Autodesk Inventor part; units mm, degrees
ref_plane "YZ Plane" through (0, 0, 0) normal (1, 0, 0) x (0, 1, 0)
ref_plane "XZ Plane" through (0, 0, 0) normal (0, 1, 0) x (-1, 0, 0)
ref_plane "XY Plane" through (0, 0, 0) normal (0, 0, 1) x (1, 0, 0)
sketch "Sketch1" plane through (0, 0, 0) normal (0, 1, 0) x (-1, 0, 0)
  line L0 (-43.5, 202.3853) -> (-0.5, 202.3853) construction
  line L1 (-0.5, 202.3853) -> (-0.5, 140.3853) construction
  line L2 (-0.5, 140.3853) -> (-43.5, 140.3853) construction
  line L3 (-43.5, 140.3853) -> (-43.5, 202.3853) construction
  line L4 (0, 112) -> (0, 260) construction
  line L5 (2.5, 205.3853) -> (-46.5, 205.3853) construction
  line L6 (-46.5, 205.3853) -> (-46.5, 137.3853) construction
  line L7 (-46.5, 137.3853) -> (2.5, 137.3853) construction
  line L8 (2.5, 137.3853) -> (2.5, 205.3853) construction
  line L9 (21.9355, 171.3853) -> (-82.4794, 171.3853) construction
  line L10 (-22, 245.5328) -> (-22, 103.5673) construction
  line L11 (-51.5, 132.3853) -> (7.5, 132.3853)
  line L12 (7.5, 132.3853) -> (7.5, 210.3853)
  line L13 (7.5, 210.3853) -> (-51.5, 210.3853)
  line L14 (-51.5, 210.3853) -> (-51.5, 132.3853)
  line L15 (-51.5, 132.3853) -> (7.5, 210.3853) construction
  line L16 (7.5, 132.3853) -> (-51.5, 210.3853) construction
  point P0 (0, 0)
  point P1 (0, 0)
  point P2 (-13.5, 205.3853)
  point P3 (-34.5, 205.3853)
  point P4 (-46.5, 183.3853)
  point P5 (-46.5, 159.3853)
  point P6 (-34.5, 137.3853)
  point P7 (-13.5, 137.3853)
  point P8 (2.5, 171.3853)
  point P9 (-22, 137.3853)
  point P10 (-22, 171.3853)
  point P11 (0, 132.3853)
  point P12 (0, 210.3853)
  point P13 (-13.5, 205.3853)
  point P14 (-34.5, 205.3853)
  point P15 (-46.5, 183.3853)
  point P16 (-46.5, 159.3853)
  point P17 (-34.5, 137.3853)
  point P18 (-13.5, 137.3853)
  point P19 (2.5, 183.3853)
  point P20 (2.5, 159.3853)
  dimension "d0" = 43
  dimension "d1" = 62
  dimension "d2" = 0.5
  dimension "d3" = 3
  dimension "d4" = 12
  dimension "d5" = 21
  dimension "d6" = 21
  dimension "d7" = 12
  dimension "d8" = 22
  dimension "d9" = 22
  dimension "d10" = 5
  dimension "d11" = 5
  dimension "d28" = 22
  dimension "d29" = 22
extrude "Extrusion1" add sketch "Sketch1" against normal blind 3
hole "Hole1" at (34.5, 0, 137.3853) at (13.5, 0, 137.3853) at (46.5, 0, 159.3853) at (46.5, 0, 183.3853) at (34.5, 0, 205.3853) at (-2.5, 0, 159.3853) at (-2.5, 0, 183.3853) at (13.5, 0, 205.3853) direction (0, -1, 0) diameter 3.2 end through all
fillet "Fillet1" radius 2 4 edges at (-7.5, -1.5, 210.3853) (51.5, -1.5, 210.3853) (51.5, -1.5, 132.3853) (-7.5, -1.5, 132.3853)
sketch "Sketch2" plane through (0, 0, 0) normal (0, 1, 0) x (1, 0, 0)
  line L0 (49.5, -132.3853) -> (-5.5, -132.3853)
  line L1 (-5.5, -210.3853) -> (49.5, -210.3853)
  line L2 (5, -132.3853) -> (43, -132.3853)
  line L3 (43, -132.3853) -> (43, -210.3853)
  line L4 (43, -210.3853) -> (5, -210.3853)
  line L5 (5, -210.3853) -> (5, -132.3853)
  arc A0 (-5.5, -132.3853) -> (-7.5, -134.3853) centre (-5.5, -134.3853) ccw
  line L6 (-7.5, -134.3853) -> (-7.5, -208.3853)
  arc A1 (-7.5, -208.3853) -> (-5.5, -210.3853) centre (-5.5, -208.3853) ccw
  line L7 (-5.5, -210.3853) -> (49.5, -210.3853)
  arc A2 (49.5, -210.3853) -> (51.5, -208.3853) centre (49.5, -208.3853) ccw
  line L8 (51.5, -208.3853) -> (51.5, -134.3853)
  arc A3 (51.5, -134.3853) -> (49.5, -132.3853) centre (49.5, -134.3853) ccw
  line L9 (49.5, -132.3853) -> (-5.5, -132.3853)
  circle A4 centre (-2.5, -183.3853) radius 1.6
  circle A5 centre (34.5, -205.3853) radius 1.6
  circle A6 centre (46.5, -159.3853) radius 1.6
  circle A7 centre (34.5, -137.3853) radius 1.6
  circle A8 centre (13.5, -137.3853) radius 1.6
  circle A9 centre (46.5, -183.3853) radius 1.6
  circle A10 centre (-2.5, -159.3853) radius 1.6
  circle A11 centre (13.5, -205.3853) radius 1.6
  line L10 (24, -128.4136) -> (24, -225.5788) construction
  point P0 (0, 0)
  point P1 (24, -132.3853)
  dimension "d31" = 38
  dimension "d32" = 10.5
  dimension "d34" = 21
extrude "Extrusion2" cut sketch "Sketch2" against normal through all contours A3 L8 A2 L1 L3 L0 | L5 L1 A1 L6 A0 L0
fillet "Fillet2" radius 2 4 edges at (5, -1.5, 210.3853) (43, -1.5, 210.3853) (43, -1.5, 132.3853) (5, -1.5, 132.3853)
equation "\"d32\" = 0.5 * d34"
properties part number "LiPo cover"
The model under review builds one solid part; all positions refer to its coordinate system, in mm. Coordinates: 2 decimals unless noted, no trailing zeros. Loops run counter-clockwise (first coordinate to the right, second up) from the corner with the lowest first, then second, coordinate; pieces in that order, holes last. Notation, with made-up numbers: (46.5, 68.5) -> (66.5, 68.5) arc R5 cw to (66.5, 77.5) -> close; hole circle Ø1 at (-14, 43.5). An arc over 180 degrees is marked (long way). Use a Markdown table: item, result. Add a question column.
1. Add section A-A on x = 34.5. Write out the cut boundary in (y, z).
2. Draft analysis for pull direction X (two halves, no side actions). For faces 1 (the face through (14.113, -1.521, 138.863)), 2 (the face through (24, -1, 210.385)), 3 (the face through (42.43, -1.521, 209.784)), state which applies: pulls with the +X half, pulls with the -X half, needs draft (parallel to the pull), parting line crosses it, or undercut.
3. To check wall thickness, follow line 1 (Z direction, x = 34.5, y = -1.7); line 2 (X direction, y = -0.8, z = 206.5); line 3 (Z direction, x = 33.5, y = -1.4). State the ranges of each line that lie inside material, in increasing order.
Returned:
| question | item | result |
|---|---|---|
| 1 | outline | (-3, 132.39) -> (0, 132.39) -> (0, 135.79) -> (-3, 135.79) -> close; (-3, 138.99) -> (0, 138.99) -> (0, 203.79) -> (-3, 203.79) -> close; (-3, 206.99) -> (0, 206.99) -> (0, 210.39) -> (-3, 210.39) -> close |
| 2 | face 1 | undercut |
| 2 | face 2 | needs draft |
| 2 | face 3 | pulls with the +X half |
| 3 | line 1 | z = 132.39 to 135.79, 138.99 to 203.79, 206.99 to 210.39 |
| 3 | line 2 | x = 5 to 12.35, 14.65 to 33.35, 35.65 to 43 |
| 3 | line 3 | z = 132.39 to 136.14, 138.63 to 204.14, 206.63 to 210.39 |
